Autodesk Inventor part; units mm, degrees
ref_plane "YZ Plane" through (0, 0, 0) normal (1, 0, 0) x (0, 1, 0)
ref_plane "XZ Plane" through (0, 0, 0) normal (0, 1, 0) x (-1, 0, 0)
ref_plane "XY Plane" through (0, 0, 0) normal (0, 0, 1) x (1, 0, 0)
sketch "Sketch1" plane through (0, 0, 0) normal (0, 0, 1) x (1, 0, 0)
  circle A0 centre (0, 0) radius 12.8905
  circle A1 centre (0, 0) radius 47.4345
  dimension "d0" = 25.781
  dimension "d1" = 94.869
extrude "Extrusion1" add sketch "Sketch1" along normal blind 3.81
sketch "Sketch2" plane through (0, 0, 3.81) normal (0, 0, 1) x (1, 0, 0)
  circle A0 centre (0, 0) radius 12.8905
  circle A1 centre (0, 0) radius 39.37
  dimension "d4" = 78.74
extrude "Extrusion2" add sketch "Sketch2" along normal blind 2.54
sketch "Sketch4" plane through (0, 0, 6.35) normal (0, 0, 1) x (1, 0, 0)
  point P0 (0, 0)
  point P1 (0, 31.75)
  point P2 (-27.4963, 15.875)
  point P3 (-27.4963, -15.875)
  point P4 (0, -31.75)
  point P5 (27.4963, -15.875)
  point P6 (27.4963, 15.875)
  dimension "d19" = 31.75
  dimension "d22" = 360
hole "Hole2" at (0, 31.75, 6.35) at (-27.4963, 15.875, 6.35) at (-27.4963, -15.875, 6.35) at (0, -31.75, 6.35) at (27.4963, -15.875, 6.35) at (27.4963, 15.875, 6.35) direction (0, 0, -1) diameter 5.5372 depth 6.35 tip angle 118 counterbore diameter 6.3246 counterbore depth 4.9378
properties part number "Worm Gear5-Bottom"
The listing builds one solid part. Answer for the finished solid, in the listing's coordinates (mm). A direction names the side the tool comes from. Round coordinates to 2 decimals unless told otherwise and drop trailing zeros. Loops run counter-clockwise (first coordinate to the right, second up) from the corner with the lowest first, then second, coordinate; pieces in that order, holes last. Notation, with made-up numbers: (-1.5, 16) - (25.5, 16) arc R20 cw to (25.5, 39) - close; hole circle Ø11 at (74.25, -25). An arc over 180 degrees is marked (long way). Return JSON: item names as keys, results as strings. Group by question number.
1. The mould has two halves that part along Y. Classify faces 3 (the flat face through (10, -10, 0)), 4 (the cylindrical face through (-31.24, 23.96, 5.06)), 5 (the cylindrical face through (29.181, -13.678, 0.696)): pulls with the +Y half, pulls with the -Y half, needs draft (parallel to the pull), parting line crosses it, or undercut.
2. The part is cut by section C-C on x = 18.5. Determine the outline of the cut face in (y, z).
3. Each of these flat-tipped pins is pushed along its axis until it touches: P1, Ø3, axis at x = 31.5, y = 27.5, coming from the +Z side; P2, Ø1.9, axis at x = 0, y = -30.5, coming from the +Z side; P3, Ø3, axis at y = -4.5, z = 1, coming from the +X side; P4, Ø1, axis at y = 4.5, z = 3, coming from the -X side. Where does it stop, or does it pass through?
4. The part is cut by section A-A on y = 0. Determine the outline of the cut face in (x, z).
5. The part is cut by section B-B on x = 0. Determine the outline of the cut face in (y, z).
6. Consider probe 1 along Y at (x, z) = (0, 4.25); probe 2 along Y at (x, z) = (0, 2.9); probe 3 along Y at (x, z) = (-25.5, 1.5). Determine where each line is inside the solid, lowest interval first.
7. The part is cut by section D-D on y = -31.75. Determine the outline of the cut face in (x, z), then the cut area to 3 significant figures.
8. Which of the six approach directions +Z, -Z, +X, -X, +Y, -Y give full straight-line access (tool end or side, diameter ignored) to faces 1 (the cylindrical face through (1.21, -34.67, 3.85)), 2 (the cylindrical face through (-6.18, -47.03, 1.88))?
Resolved:
{
 "1": {"face 3": "needs draft", "face 4": "parting line crosses it", "face 5": "undercut"},
 "2": {"outline": "(-43.68, 0) - (43.68, 0) - (43.68, 3.81) - (34.75, 3.81) - (34.75, 6.35) - (-34.75, 6.35) - (-34.75, 3.81) - (-43.68, 3.81) - close"},
 "3": {"P1": "stops at z = 3.81", "P2": "passes through", "P3": "stops at x = 47.34", "P4": "stops at x = -47.27"},
 "4": {"outline": "(-47.43, 0) - (-12.89, 0) - (-12.89, 6.35) - (-39.37, 6.35) - (-39.37, 3.81) - (-47.43, 3.81) - close; (12.89, 0) - (47.43, 0) - (47.43, 3.81) - (39.37, 3.81) - (39.37, 6.35) - (12.89, 6.35) - close"},
 "5": {"outline": "(-47.43, 0) - (-34.52, 0) - (-34.52, 1.41) - (-34.91, 1.41) - (-34.91, 6.35) - (-39.37, 6.35) - (-39.37, 3.81) - (-47.43, 3.81) - close; (-28.98, 0) - (-12.89, 0) - (-12.89, 6.35) - (-28.59, 6.35) - (-28.59, 1.41) - (-28.98, 1.41) - close; (12.89, 0) - (28.98, 0) - (28.98, 1.41) - (28.59, 1.41) - (28.59, 6.35) - (12.89, 6.35) - close; (34.52, 0) - (47.43, 0) - (47.43, 3.81) - (39.37, 3.81) - (39.37, 6.35) - (34.91, 6.35) - (34.91, 1.41) - (34.52, 1.41) - close"},
 "6": {"probe 1": "y = -39.37 to -34.91, -28.59 to -12.89, 12.89 to 28.59, 34.91 to 39.37", "probe 2": "y = -47.43 to -34.91, -28.59 to -12.89, 12.89 to 28.59, 34.91 to 47.43", "probe 3": "y = -40 to -18.33, -13.42 to 13.42, 18.33 to 40"},
 "7": {"outline": "(-35.24, 0) - (-2.77, 0) - (-2.77, 1.41) - (-3.16, 1.41) - (-3.16, 6.35) - (-23.28, 6.35) - (-23.28, 3.81) - (-35.24, 3.81) - close; (2.77, 0) - (35.24, 0) - (35.24, 3.81) - (23.28, 3.81) - (23.28, 6.35) - (3.16, 6.35) - (3.16, 1.41) - (2.77, 1.41) - close", "area": "348 mm²"},
 "8": {"face 1": "+Z", "face 2": "+Z, -Z"}
}
